```python
from build123d import *

# Parameters (mm, degrees)
SKETCH1_R           = 15
SKETCH1_R_2         = 14
BOSS_EXTRUDE1_DEPTH = 220
SKETCH2_R           = 3
CUT_EXTRUDE1_DEPTH  = 15


with BuildPart() as part:
    # Sketch1 → Boss-Extrude1 (new body)
    with BuildSketch(Plane(origin=(0, 0, 0), x_dir=(1, 0, 0), z_dir=(0, 1, 0))):
        with Locations(Location((0, 0, 0), (0, 0, 270))):
            Circle(SKETCH1_R)
        with Locations(Location((0, 0, 0), (0, 0, 270))):
            Circle(SKETCH1_R_2, mode=Mode.SUBTRACT)
    extrude(amount=BOSS_EXTRUDE1_DEPTH)

    # Sketch2 → Cut-Extrude1 (cut, symmetric)
    with BuildSketch(Plane.XY):
        with Locations((0, 200)):
            Circle(SKETCH2_R)
        with Locations((0, 20)):
            Circle(SKETCH2_R)
    extrude(amount=CUT_EXTRUDE1_DEPTH, both=True, mode=Mode.SUBTRACT)


solid = part.part
```
Geometry check sheet. Reference: the model listing, model coordinates, mm. Coordinates: 2 decimals unless noted, no trailing zeros. Order: outer loops, then holes, each group sorted by start corner. A loop starts at its lowest first (then second) coordinate and runs counter-clockwise, first axis right, second up. Notation, with made-up numbers: (57.5, 43) - (67.5, 43) arc R13 cw to (67.5, 47) - close; hole circle Ø3 at (16.5, -22). An arc over 180 degrees is marked (long way). Use one line per item in the form item = value.
1. Section check B-B (z = 0). Record the boundary of the cut face in (x, y), then the cut area to 3 significant figures.
Here are the results:
outline = (-15, 0) - (-14, 0) - (-14, 220) - (-15, 220) - close; (14, 0) - (15, 0) - (15, 220) - (14, 220) - close
area = 440 mm²
2. Gauge pin test, flat ends, axial feed: pin 1 (6 mm diameter, centred on x = -8, y = 52.5, fed in from -Z); pin 2 (5.5 mm diameter, centred on x = 0, y = 20, fed in from -Z); pin 3 (4 mm diameter, centred on x = 9.5, y = 104.5, fed in from -Z); pin 4 (5 mm diameter, centred on y = 90.5, z = 10.5, fed in from -X). Record the tip position at first contact, or that the pin passes through.
Here are the results:
pin_1 = -14.14
pin_2 = through
pin_3 = -12.99
pin_4 = -12.69
3. Draft check along Y on faces 1 (the face through (-2.4, 198.2, 14.3)), 2 (the face through (-13.67, 108.46, -3.03)). Enter one of: pulls with the +Y half, pulls with the -Y half, needs draft (parallel to the pull), parting line crosses it, or undercut.
Here are the results:
face_1 = undercut
face_2 = needs draft
4. Section check A-A (x = 0). Record the boundary of the cut face in (y, z).
Here are the results:
outline = (0, -15) - (17, -15) - (17, -14) - (0, -14) - close; (0, 14) - (17, 14) - (17, 15) - (0, 15) - close; (23, -15) - (197, -15) - (197, -14) - (23, -14) - close; (23, 14) - (197, 14) - (197, 15) - (23, 15) - close; (203, -15) - (220, -15) - (220, -14) - (203, -14) - close; (203, 14) - (220, 14) - (220, 15) - (203, 15) - close
5. Scan lines: line 1 (Z direction, x = -0.5, y = 41); line 2 (X direction, y = 71, z = 0); line 3 (Z direction, x = 8.5, y = 192). Record each from-to range of solid material in increasing order.
Here are the results:
line_1 = -14.99 to -13.99, 13.99 to 14.99
line_2 = -15 to -14, 14 to 15
line_3 = -12.36 to -11.12, 11.12 to 12.36
6. Section check D-D (y = 69.5). Record the boundary of the cut face in (x, z), then the cut area to 3 significant figures.
Here are the results:
outline = circle Ø30 at (0, 0); hole circle Ø28 at (0, 0)
area = 91.1 mm²
